Input: part model. Units: mm. Frame: model coordinates. Face numbers are marked on the shaded views. A direction names the side the tool comes from. Give positions to 0.01 mm unless a question says otherwise; leave off trailing zeros. Loops run counter-clockwise (first coordinate to the right, second up) from the corner with the lowest first, then second, coordinate; pieces in that order, holes last. Notation, with made-up numbers: (-11.5, 52) - (17.5, 52) arc R16 cw to (17.5, 78) - close; hole circle Ø6 at (-23.75, -27). An arc over 180 degrees is marked (long way). Answer as a JSON object with one key per item and string values.
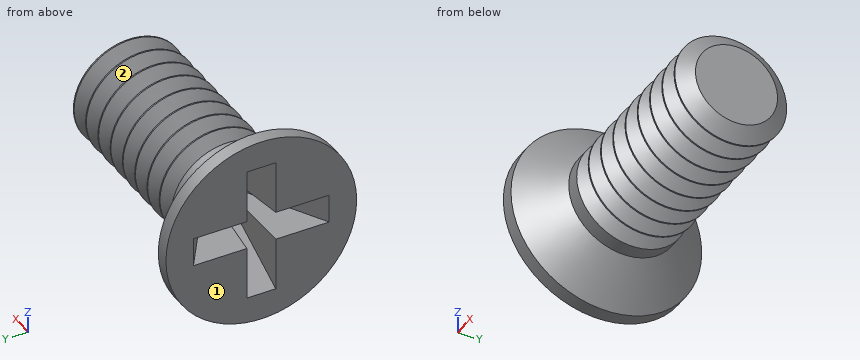
from build123d import *

# Parameters (mm, degrees)
SKETCH3_W         = 0.7366
SKETCH3_H         = 3.4544
SKETCH4_W         = 0.3683
SKETCH4_H         = 0.3683
CIRPATTERN1_COUNT = 2
CIRPATTERN1_ANGLE = 90
THDSCHPAT_COUNT   = 9
THDSCHPAT_PITCH   = 0.56515


with BuildPart() as part:
    # BodySke → Base-Revolve (revolve)
    with BuildSketch(Plane.XY):
        Polygon((0, 0), (0, 2.4257), (0.35193134, 2.4257), (1.1938, 1.4224), (6.35, 1.4224), (6.35, 0), align=None)
    revolve(axis=Axis((-6.35, 0, 0), (1, 0, 0)))

    # Sketch3 → Cross section 0
    with BuildSketch(Plane.ZY):
        Rectangle(SKETCH3_W, SKETCH3_H)
    # Sketch4 → Cross section 1
    with BuildSketch(Plane.ZY.offset(-2.2606)):
        Rectangle(SKETCH4_W, SKETCH4_H)
    cross = loft(mode=Mode.SUBTRACT)

    # CirPattern1: Cross ×2 about axis
    cirpattern1_axis = Axis((0, 0, 0), (1, 0, 0))
    for i in range(1, CIRPATTERN1_COUNT):
        add(cross.rotate(cirpattern1_axis, i * CIRPATTERN1_ANGLE / (CIRPATTERN1_COUNT - 1)), mode=Mode.SUBTRACT)

    # ThdSchSke → ThreadSchematic (revolve, cut)
    with BuildSketch(Plane.XY):
        Polygon((1.8288254, -1.04394), (1.563824855, -1.4224), (1.563824855, -1.778), (2.093825945, -1.778), (2.093825945, -1.4224), align=None)
    threadschematic = revolve(axis=Axis((-3.175, 0, 0), (1, 0, 0)), mode=Mode.SUBTRACT)

    # ThdSchPat: ThreadSchematic ×9
    with Locations(*[(i * THDSCHPAT_PITCH, 0, 0) for i in range(1, THDSCHPAT_COUNT)]):
        add(threadschematic, mode=Mode.SUBTRACT)


solid = part.part
Item 1: Cut plane C-C (x = 4). Return loops of the section in (y, z), then the cut area to 3 significant figures.
Geometry check:
{"outline": "circle Ø2.34 at (0, 0)", "area": "4.31 mm2"}
Item 2: Contact query for flat-ended pins moving along their axis: P1, Ø1.5, axis at x = 2, z = 0, coming from the -Y side; P2, Ø2, axis at x = 3.5, y = 0, coming from the +Z side. Output: stop coordinate, or through.
Geometry check:
{"P1": "stops at y = -1.42", "P2": "stops at z = 1.42"}
Item 3: Cut plane B-B (y = -1.3). Give the number of separate pieces and of enclosed holes in the cut face, then the cut area to 3 significant figures.
Geometry check:
{"separate pieces": "9", "enclosed holes": "0", "area": "5.21 mm2"}
Item 4: Access query for the marked faces 1 and 2. Directions: +Z, -Z, +X, -X, +Y, -Y. A direction counts if a zero-diameter tool reaches every point of the face in a straight line with its end or side. Return the directions, or none.
Geometry check:
{"face 1": "+Z, -Z, -X, +Y, -Y", "face 2": "none"}
Item 5: Material intervals for line 1 (Y direction, x = 1.25, z = 0.6); line 2 (Y direction, x = 1.5, z = -1.1); line 3 (Z direction, x = 3.75, y = -0.5), sorted ascending. Write a range as [from, to].
Geometry check:
{"line 1": "y = [-1.29, -0.27], [0.27, 1.29]", "line 2": "y = [-0.9, 0.9]", "line 3": "z = [-1.27, 1.27]"}
Item 6: Cut plane A-A (x = 2.5). Return loops of the section in (y, z), then the cut area to 3 significant figures.
Geometry check:
{"outline": "circle Ø2.39 at (0, 0)", "area": "4.49 mm2"}
